```python
from build123d import *

# Parameters (mm, degrees)
SKETCH026_W             = 42.3
SKETCH026_H             = 42.3
PAD008_DEPTH            = 40
SKETCH025_R             = 11
PAD009_DEPTH            = 3
SKETCH023_R             = 5.1
PAD010_DEPTH            = 21
SKETCH027_R             = 1.5
POCKET012_DEPTH         = 5
CHAMFER002_SIZE         = 5
BODY007_PLACEMENT_ANGLE = 90


with BuildPart() as part:
    # Sketch026 → Pad008 (new body)
    with BuildSketch(Plane.XY):
        Rectangle(SKETCH026_W, SKETCH026_H)
    extrude(amount=PAD008_DEPTH)

    # Sketch025 (on Face6 of Pad008) → Pad009 (join)
    with BuildSketch(Plane.XY.offset(40)):
        Circle(SKETCH025_R)
    extrude(amount=PAD009_DEPTH)

    # Sketch023 (on Face8 of Pad009) → Pad010 (join)
    with BuildSketch(Plane.XY.offset(43)):
        Circle(SKETCH023_R)
    extrude(amount=PAD010_DEPTH)

    # Sketch027 (on Face5 of Pad010) → Pocket012 (cut)
    with BuildSketch(Plane.XY.offset(40)):
        with Locations((-15.5, 15.5)):
            Circle(SKETCH027_R)
        with Locations((15.5, 15.5)):
            Circle(SKETCH027_R)
        with Locations((15.5, -15.5)):
            Circle(SKETCH027_R)
        with Locations((-15.5, -15.5)):
            Circle(SKETCH027_R)
    extrude(amount=-POCKET012_DEPTH, mode=Mode.SUBTRACT)

    # Chamfer002
    chamfer002_edges = [part.edges().sort_by_distance(p)[0] for p in [
        (21.15, 21.15, 20),
        (21.15, -21.15, 20),
        (-21.15, 21.15, 20),
        (-21.15, -21.15, 20),
    ]]
    chamfer(chamfer002_edges, length=CHAMFER002_SIZE)


with BuildPart() as part_1:
    # Body007 placement: moved
    add(part.part.moved(Location((159, 0.1, 21.25))).rotate(Axis((159, 0.1, 21.25), (0, -1, 0)), BODY007_PLACEMENT_ANGLE))


solid = part_1.part
```
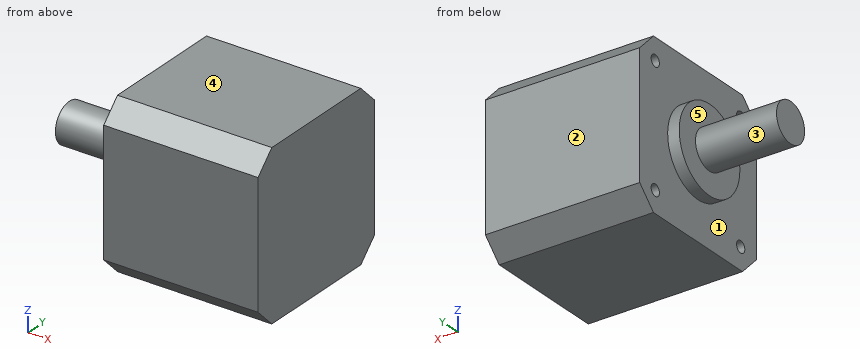
Source: CAD feature listing. Evaluate the final solid. Frame: model axes, mm. Face numbers are marked on the shaded views. A direction names the side the tool comes from. Round coordinates to 2 decimals unless told otherwise and drop trailing zeros. Order: outer loops, then holes, each group sorted by start corner. A loop starts at its lowest first (then second) coordinate and runs counter-clockwise, first axis right, second up. Notation, with made-up numbers: (16, 23) -> (31, 23) arc R4 cw to (31, 29) -> close; hole circle Ø3 at (12, 1.25). An arc over 180 degrees is marked (long way). Use CSV: the item, a comma, the result in double quotes.
(1) Section C-C on x = 143.5. Return the cut outline in (y, z).
Report:
outline,"(-21.05, 5.1) -> (-16.05, 0.1) -> (16.25, 0.1) -> (21.25, 5.1) -> (21.25, 37.4) -> (16.25, 42.4) -> (-16.05, 42.4) -> (-21.05, 37.4) -> close"
(2) Section D-D on y = -4. Return the cut outline in (x, z), and give its area (3 significant figures).
Report:
outline,"(95, 18.22) -> (116, 18.22) -> (116, 11.04) -> (119, 11.04) -> (119, 0.1) -> (159, 0.1) -> (159, 42.4) -> (119, 42.4) -> (119, 31.46) -> (116, 31.46) -> (116, 24.28) -> (95, 24.28) -> close"
area,"1,880 mm^2"
(3) Section A-A on x = 123. Return the cut outline in (y, z), and give its area (3 significant figures).
Report:
outline,"(-21.05, 5.1) -> (-16.05, 0.1) -> (16.25, 0.1) -> (21.25, 5.1) -> (21.25, 37.4) -> (16.25, 42.4) -> (-16.05, 42.4) -> (-21.05, 37.4) -> close; hole circle Ø3 at (-15.4, 5.75); hole circle Ø3 at (-15.4, 36.75); hole circle Ø3 at (15.6, 5.75); hole circle Ø3 at (15.6, 36.75)"
area,"1,710 mm^2"
(4) Pull-direction query (Z, two-part tool) for the marked faces 3, 4 and 5; classes: +Z half, -Z half, draft (parallel to the pull), parting line (faces both ways), or undercut.
Report:
face 3,"parting line"
face 4,"+Z half"
face 5,"draft"
(5) First-contact query: pin 1 Ø4 at (y, z) = (-15.4, 36.75) entering from -X; pin 2 Ø0.9 at (y, z) = (-16, 37.5) entering from -X; pin 3 Ø5 at (y, z) = (5.5, 12.5) entering from -X. Flat tips, straight axial feed; report the tip coordinate or a pass-through.
Report:
pin 1,"x = 119"
pin 2,"x = 124"
pin 3,"x = 116"
(6) Ray query, L1, parallel to Y at x = 122.3, z = 5.75; L2, parallel to Z at x = 122, y = -15; L3, parallel to X at y = -7.5, z = 35. Return the intervals inside material, ascending.
Report:
L1,"-21.05 to -16.9, -13.9 to 14.1, 17.1 to 21.25"
L2,"0.1 to 4.3, 7.2 to 35.3, 38.2 to 42.4"
L3,"119 to 159"
(7) Section B-B on z = 21.25. Return the cut outline in (x, y), and give its area (3 significant figures).
Report:
outline,"(95, -5) -> (116, -5) -> (116, -10.9) -> (119, -10.9) -> (119, -21.05) -> (159, -21.05) -> (159, 21.25) -> (119, 21.25) -> (119, 11.1) -> (116, 11.1) -> (116, 5.2) -> (95, 5.2) -> close"
area,"1,970 mm^2"
(8) Access query for the marked faces 1 and 2. Directions: +Z, -Z, +X, -X, +Y, -Y. A direction counts if a zero-diameter tool reaches every point of the face in a straight line with its end or side. Return the directions, or none.
Report:
face 1,"-X"
face 2,"+Z, -Z, +X, -X, +Y"
